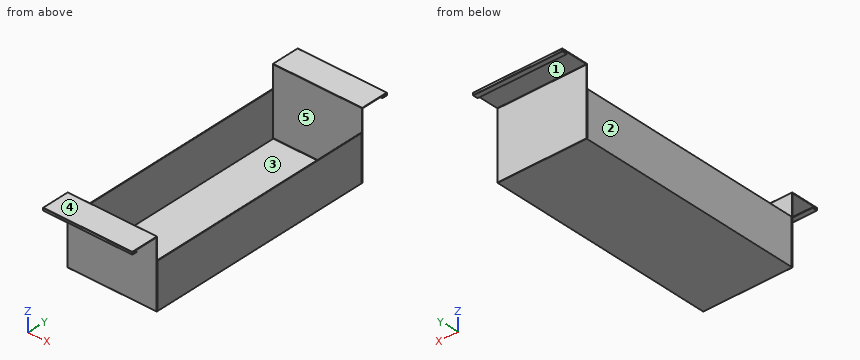
from build123d import *

# Parameters (mm, degrees)
F1_DEPTH = 200
F2_W     = 1.5
F2_H     = 515
F3_DEPTH = 100


with BuildPart() as f1:
    # F0 (on Right) → F1 (new body)
    with BuildSketch(Plane.YZ):
        with BuildLine():
            Line((-304.685603, 141.559852), (-304.685603, 143.059852))
            Line((-304.685603, 143.059852), (-313.685603, 143.059852))
            ThreePointArc((-313.685603, 143.059852), (-314.39271, 143.352745), (-314.685603, 144.059852))
            Line((-314.685603, 144.059852), (-314.685603, 145.059852))
            ThreePointArc((-314.685603, 145.059852), (-314.39271, 145.766959), (-313.685603, 146.059852))
            Line((-313.685603, 146.059852), (-255.685603, 146.059852))
            ThreePointArc((-255.685603, 146.059852), (-254.978496, 145.766959), (-254.685603, 145.059852))
            Line((-254.685603, 145.059852), (-254.685603, -2.940148))
            ThreePointArc((-254.685603, -2.940148), (-254.39271, -3.647255), (-253.685603, -3.940148))
            Line((-253.685603, -3.940148), (264.314397, -3.940148))
            ThreePointArc((264.314397, -3.940148), (265.021504, -3.647255), (265.314397, -2.940148))
            Line((265.314397, -2.940148), (265.314397, 145.059852))
            ThreePointArc((265.314397, 145.059852), (265.60729, 145.766959), (266.314397, 146.059852))
            Line((266.314397, 146.059852), (324.314397, 146.059852))
            ThreePointArc((324.314397, 146.059852), (325.021504, 145.766959), (325.314397, 145.059852))
            Line((325.314397, 145.059852), (325.314397, 144.059852))
            ThreePointArc((325.314397, 144.059852), (325.021504, 143.352745), (324.314397, 143.059852))
            Line((324.314397, 143.059852), (315.314397, 143.059852))
            Line((315.314397, 143.059852), (315.314397, 141.559852))
            Line((315.314397, 141.559852), (325.814397, 141.559852))
            ThreePointArc((325.814397, 141.559852), (326.521504, 141.852745), (326.814397, 142.559852))
            Line((326.814397, 142.559852), (326.814397, 146.559852))
            ThreePointArc((326.814397, 146.559852), (326.521504, 147.266959), (325.814397, 147.559852))
            Line((325.814397, 147.559852), (264.814397, 147.559852))
            ThreePointArc((264.814397, 147.559852), (264.10729, 147.266959), (263.814397, 146.559852))
            Line((263.814397, 146.559852), (263.814397, -1.440148))
            ThreePointArc((263.814397, -1.440148), (263.521504, -2.147255), (262.814397, -2.440148))
            Line((262.814397, -2.440148), (-252.185603, -2.440148))
            ThreePointArc((-252.185603, -2.440148), (-252.89271, -2.147255), (-253.185603, -1.440148))
            Line((-253.185603, -1.440148), (-253.185603, 146.559852))
            ThreePointArc((-253.185603, 146.559852), (-253.478496, 147.266959), (-254.185603, 147.559852))
            Line((-254.185603, 147.559852), (-315.185603, 147.559852))
            ThreePointArc((-315.185603, 147.559852), (-315.89271, 147.266959), (-316.185603, 146.559852))
            Line((-316.185603, 146.559852), (-316.185603, 142.559852))
            ThreePointArc((-316.185603, 142.559852), (-315.89271, 141.852745), (-315.185603, 141.559852))
            Line((-315.185603, 141.559852), (-304.685603, 141.559852))
        make_face()
    extrude(amount=-F1_DEPTH)

    # F2 (on face) → F3 (join)
    with BuildSketch(Plane.XY.offset(-2.440148)):
        with Locations((-0.75, 5.314397)):
            Rectangle(F2_W, F2_H)
        with Locations((-199.25, 5.314397)):
            Rectangle(F2_W, F2_H)
    extrude(amount=F3_DEPTH)


solid = f1.part
Verification items for the finished model (mm, model axes). Face numbers are marked on the shaded views. A direction names the side the tool comes from. Give positions to 0.01 mm unless a question says otherwise; leave off trailing zeros. Loops run counter-clockwise (first coordinate to the right, second up) from the corner with the lowest first, then second, coordinate; pieces in that order, holes last. Notation, with made-up numbers: (18, 41) - (26, 41) arc R18 ccw to (26, 66) - close; hole circle Ø8 at (84, 65). An arc over 180 degrees is marked (long way). Write item = value, one per line. Start each with the question number.
Q1. Cross-section at A-A, the plane z = 85. Enter the section's corners in (x, y).
Q2. Tool access check on the marked faces 3, 4 and 5. Record the directions out of +Z, -Z, +X, -X, +Y, -Y that give a thin tool (end or side, any length) a straight path to the whole face; none if there is none.
Q3. Cross-section at B-B, the plane y = -207. Enter the section's corners in (x, z).
Q4. Depth check by flat-ended pin: P1, Ø5, axis at x = -133, y = 321, coming from the -Z side; P2, Ø5, axis at x = -100, z = 37, coming from the +Y side; P3, Ø10, axis at y = 70.5, z = 15, coming from the +X side; P4, Ø4, axis at x = -73.5, y = 161, coming from the +Z side. Enter the tip coordinate at first touch or a pass-through.
Q5. Mould release check, pull along Y, two halves, no side actions. Record for the marked faces 1 and 2: released by +Y, released by -Y, zero draft, split by the parting line, or undercut.
Q6. Thickness scan on line 1 (Y direction, x = -180, z = 80.5); line 2 (X direction, y = -135.5, z = 77.5); line 3 (Z direction, x = -11, y = -88). Record the ranges inside material, lowest first.
Answer key:
q1.outline = (-200, -254.69) - (0, -254.69) - (0, -253.19) - (-200, -253.19) - close; (-200, -252.19) - (-198.5, -252.19) - (-198.5, 262.81) - (-200, 262.81) - close; (-200, 263.81) - (0, 263.81) - (0, 265.31) - (-200, 265.31) - close; (-1.5, -252.19) - (0, -252.19) - (0, 262.81) - (-1.5, 262.81) - close
q2.face_3 = +Z
q2.face_4 = +Z, +X, -X, +Y, -Y
q2.face_5 = +Z, +X, -X
q3.outline = (-200, -3.94) - (0, -3.94) - (0, 97.56) - (-1.5, 97.56) - (-1.5, -2.44) - (-198.5, -2.44) - (-198.5, 97.56) - (-200, 97.56) - close
q4.P1 = 141.56
q4.P2 = 265.31
q4.P3 = 0
q4.P4 = -2.44
q5.face_1 = undercut
q5.face_2 = zero draft
q6.line_1 = -254.69 to -253.19, 263.81 to 265.31
q6.line_2 = -200 to -198.5, -1.5 to 0
q6.line_3 = -3.94 to -2.44
